Could you check a few things on this drawing? It's one solid part, dimensions in mm from its lowest x, y, z. Give positions to 0.01 mm unless a question says otherwise; leave off trailing zeros. Loops run counter-clockwise (first coordinate to the right, second up) from the corner with the lowest first, then second, coordinate; pieces in that order, holes last. Notation, with made-up numbers: M 51.5,-15.75 L 69.5,-15.75 A20 ccw 69.5,23.25 Z; hole C 63,-2.75 d6. An arc over 180 degrees is marked long. Return JSON: item names as keys, results as strings. Group by question number.
1. If we section it at C-C (x = 14.5): Write out the boundary of the cut face in (y, z), plus the area to 3 significant figures.
2. For pin 1 (1.1 mm diameter, centred on x = 15.5, z = 40.5, fed in from +Y); pin 2 (6 mm diameter, centred on y = 13, z = 32.5, fed in from -X); pin 3 (6 mm diameter, centred on x = 10, y = 10, fed in from -Z); pin 4 (0.5 mm diameter, centred on x = 8, z = 40.5, fed in from -Y), each with a flat end and sliding along its axis, tell me the tip position at first contact or that it passes through.
3. If we mould it in two halves opening along X, with no side actions, what happens to the marked faces 1, 2 and 3? For each: +X half, -X half, draft (parallel to the pull), parting line (faces both ways), or undercut.
4. If we section it at B-B (y = 10): Write out the boundary of the cut face in (x, z), plus the area to 3 significant figures.
5. Please list where these lines run through material, in increasing order: line 1 (Y direction, x = 10, z = 13); line 2 (Z direction, x = 4.25, y = 18); line 3 (X direction, y = 1.5, z = 38).
6. If we section it at A-A (x = 10): Write out the boundary of the cut face in (y, z).
7. If we section it at D-D (z = 3.5): Write out the boundary of the cut face in (x, y).
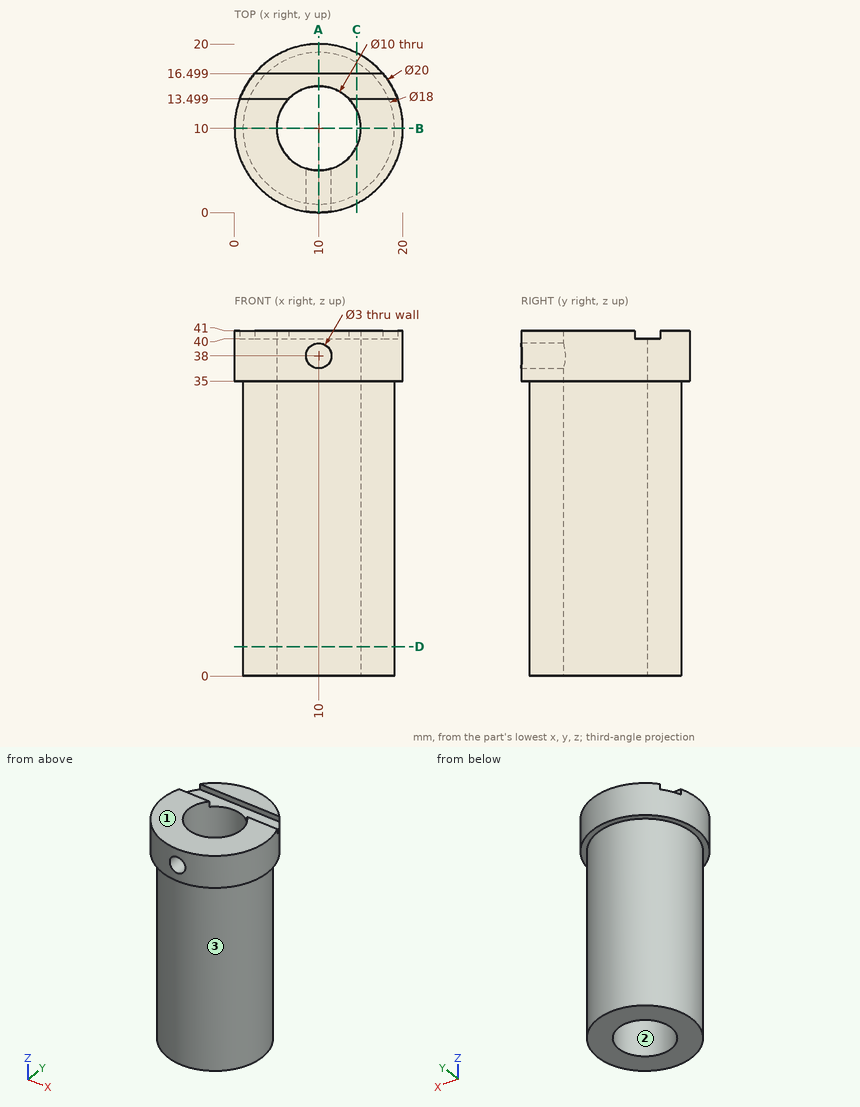
Answer:
{
 "1": {"outline": "M 1.07,35 L 2.21,35 L 2.21,0 L 7.82,0 L 7.82,41 L 1.07,41 Z; M 12.18,0 L 17.79,0 L 17.79,35 L 18.93,35 L 18.93,41 L 16.5,41 L 16.5,40 L 13.5,40 L 13.5,41 L 12.18,41 Z", "area": "471 mm²"},
 "2": {"pin 1": "stops at y = 18.69", "pin 2": "stops at x = 0.09", "pin 3": "passes through", "pin 4": "stops at y = 0.15"},
 "3": {"face 1": "draft", "face 2": "undercut", "face 3": "parting line"},
 "4": {"outline": "M 0,35 L 1,35 L 1,0 L 5,0 L 5,41 L 0,41 Z; M 15,0 L 19,0 L 19,35 L 20,35 L 20,41 L 15,41 Z", "area": "340 mm²"},
 "5": {"line 1": "y = 1 to 5, 15 to 19", "line 2": "z = 35 to 41", "line 3": "x = 4.73 to 8.5, 11.5 to 15.27"},
 "6": {"outline": "M 0,35 L 1,35 L 1,0 L 5,0 L 5,36.5 L 0,36.5 Z; M 0,39.5 L 5,39.5 L 5,41 L 0,41 Z; M 15,0 L 19,0 L 19,35 L 20,35 L 20,41 L 16.5,41 L 16.5,40 L 15,40 Z"},
 "7": {"outline": "C 10,10 d18; hole C 10,10 d10"}
}
